```python
from build123d import *

# Parameters (mm, degrees)
SKETCH_1_R          = 3.5
SKETCH_1_R_2        = 3
EXTRUDE_1_DEPTH     = 10
SKETCH_2_R          = 20
EXTRUDE_2_DEPTH     = 16
EXTRUDE_2_DRAFT     = -5
SKETCH_4_W          = 48
SKETCH_4_H          = 48
CUT_EXTRUDE_1_DEPTH = 16
EXTRUDE_3_DEPTH     = 2
EXTRUDE_3_DRAFT     = -10


with BuildPart() as part:
    # Sketch 1 → Extrude 1 (new body)
    with BuildSketch(Plane(origin=(0, 0, 0), x_dir=(1, 0, 0), z_dir=(0, 1, 0))):
        with BuildLine():
            Line((0, -20), (69, -20))
            ThreePointArc((69, -20), (73.242640687, -18.242640687), (75, -14))
            Line((75, -14), (75, 37))
            Line((75, 37), (37, 75))
            Line((37, 75), (-14, 75))
            ThreePointArc((-14, 75), (-18.242640687, 73.242640687), (-20, 69))
            Line((-20, 69), (-20, 0))
            ThreePointArc((-20, 0), (-14.142135624, -14.142135624), (0, -20))
        make_face()
        with Locations(Location((65, -5, 0), (0, 0, 270))):
            Circle(SKETCH_1_R, mode=Mode.SUBTRACT)
        with Locations(Location((55, -10, 0), (0, 0, 270))):
            Circle(SKETCH_1_R_2, mode=Mode.SUBTRACT)
        with Locations(Location((30, -5, 0), (0, 0, 270))):
            Circle(SKETCH_1_R, mode=Mode.SUBTRACT)
        with Locations(Location((25, -10, 0), (0, 0, 270))):
            Circle(SKETCH_1_R_2, mode=Mode.SUBTRACT)
        with Locations(Location((-5, 30, 0), (0, 0, 270))):
            Circle(SKETCH_1_R, mode=Mode.SUBTRACT)
        with Locations(Location((-5, 65, 0), (0, 0, 270))):
            Circle(SKETCH_1_R, mode=Mode.SUBTRACT)
        with Locations(Location((-10, 25, 0), (0, 0, 270))):
            Circle(SKETCH_1_R_2, mode=Mode.SUBTRACT)
        with Locations(Location((-10, 55, 0), (0, 0, 270))):
            Circle(SKETCH_1_R_2, mode=Mode.SUBTRACT)
    extrude(amount=-EXTRUDE_1_DEPTH)


with BuildPart() as extrude_2_tool:
    # Sketch 2 → Extrude 2 (with draft: the straight prism first)
    with BuildSketch(Plane(origin=(0, -10, 0), x_dir=(1, 0, 0), z_dir=(0, 1, 0))):
        Circle(SKETCH_2_R)
    extrude(amount=-EXTRUDE_2_DEPTH)
    # Extrude 2: the draft: its side faces are tilted about the plane it starts from
    extrude_2_sides = [extrude_2_tool.faces().sort_by_distance(p)[0] for p in [
        (-20, -18, 0),
    ]]
    draft(extrude_2_sides, Plane(origin=(0, -10, 0), x_dir=(1, 0, 0), z_dir=(0, 1, 0)), EXTRUDE_2_DRAFT)


with BuildPart() as part_1:
    add(part.part)

    # Extrude 2: add extrude_2_tool
    add(extrude_2_tool.part)

    # Sketch 3 → Revolve 1 (revolve)
    with BuildSketch(Plane.XY, mode=Mode.PRIVATE) as revolve_1_sk:
        Polygon((0, -26), (12, -26), (14.4, -26.643078062), (14.4, -33.356921938), (12, -34), (0, -34), align=None)
    revolve(revolve_1_sk.sketch.rotate(Axis((0, -34, 0), (0, 1, 0)), 270), axis=Axis((0, -34, 0), (0, 1, 0)))

    # Sketch 4 → Cut-Extrude 1 (cut)
    with BuildSketch(Plane(origin=(0, -26, 0), x_dir=(1, 0, 0), z_dir=(0, 1, 0))):
        Rectangle(SKETCH_4_W, SKETCH_4_H)
        Polygon((-12, -6.92820323), (0, -13.856406461), (12, -6.92820323), (12, 6.92820323), (0, 13.856406461), (-12, 6.92820323), align=None, mode=Mode.SUBTRACT)
    extrude(amount=-CUT_EXTRUDE_1_DEPTH, mode=Mode.SUBTRACT)

    # Sketch 5 → Cut-Revolve 1 (revolve, cut)
    with BuildSketch(Plane.XY, mode=Mode.PRIVATE) as cut_revolve_1_sk:
        Polygon((0, 0), (8, 0), (6.9175, -1.0825), (6.9175, -32.9175), (8, -34), (0, -34), align=None)
    revolve(cut_revolve_1_sk.sketch.rotate(Axis((0, -34, 0), (0, 1, 0)), 270), axis=Axis((0, -34, 0), (0, 1, 0)), mode=Mode.SUBTRACT)


with BuildPart() as extrude_3_tool:
    # Sketch 6 → Extrude 3 (with draft: the straight prism first)
    with BuildSketch(Plane(origin=(0, -10, 0), x_dir=(1, 0, 0), z_dir=(0, 1, 0))):
        with BuildLine():
            Line((6.573950263, 34.573950263), (34.573950263, 6.573950263))
            ThreePointArc((34.573950263, 6.573950263), (38.109484168, 5.109484168), (41.645018074, 6.573950263))
            Line((41.645018074, 6.573950263), (69.929289322, 34.85822151))
            ThreePointArc((69.929289322, 34.85822151), (71.393755416, 38.393755416), (69.929289322, 41.929289322))
            Line((69.929289322, 41.929289322), (41.929289322, 69.929289322))
            ThreePointArc((41.929289322, 69.929289322), (38.393755416, 71.393755416), (34.85822151, 69.929289322))
            Line((34.85822151, 69.929289322), (6.573950263, 41.645018074))
            ThreePointArc((6.573950263, 41.645018074), (5.109484168, 38.109484168), (6.573950263, 34.573950263))
        make_face()
    extrude(amount=-EXTRUDE_3_DEPTH)
    # Extrude 3: the draft: its side faces are tilted about the plane it starts from
    extrude_3_sides = [extrude_3_tool.faces().sort_by_distance(p)[0] for p in [
        (20.573950263, -11, -20.573950263),
        (38.109484168, -11, -5.109484168),
        (55.787153698, -11, -20.716085886),
        (71.393755416, -11, -38.393755416),
        (55.929289322, -11, -55.929289322),
        (38.393755416, -11, -71.393755416),
        (20.716085886, -11, -55.787153698),
        (5.109484168, -11, -38.109484168),
    ]]
    draft(extrude_3_sides, Plane(origin=(0, -10, 0), x_dir=(1, 0, 0), z_dir=(0, 1, 0)), EXTRUDE_3_DRAFT)


with BuildPart() as part_2:
    add(part_1.part)

    # Extrude 3: add extrude_3_tool
    add(extrude_3_tool.part)

    # Sketch 7 → Revolve 2 (revolve)
    with BuildSketch(Plane(origin=(0, 0, 0), x_dir=(0.7071067811865476, 0, -0.7071067811865475), z_dir=(0.7071067811865475, 0, 0.7071067811865476)), mode=Mode.PRIVATE) as revolve_2_sk:
        with BuildLine():
            Line((55, -12), (75, -12))
            Line((75, -12), (72.585786438, -14.414213562))
            ThreePointArc((72.585786438, -14.414213562), (71.93693974, -14.847759065), (71.171572875, -15))
            Line((71.171572875, -15), (55, -15))
            Line((55, -15), (55, -12))
        make_face()
    revolve(revolve_2_sk.sketch.rotate(Axis((38.890872965, -15, -38.890872965), (0, 1, 0)), 225), axis=Axis((38.890872965, -15, -38.890872965), (0, 1, 0)))


solid = part_2.part
```
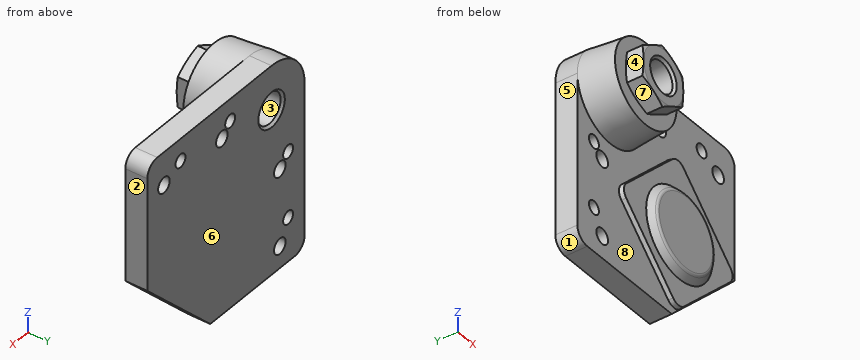
Read the model definition and answer for the solid it produces. Units are mm, in the model's axes. Face numbers are marked on the shaded views. A direction names the side the tool comes from. Round coordinates to 2 decimals unless told otherwise and drop trailing zeros. Loops run counter-clockwise (first coordinate to the right, second up) from the corner with the lowest first, then second, coordinate; pieces in that order, holes last. Notation, with made-up numbers: (14, -6.5) -> (18, -6.5) arc R17 cw to (18, -2.5) -> close; hole circle Ø11 at (75, 36.25). An arc over 180 degrees is marked (long way). One line per item, written item: value.
1) For the marked faces 4, 5, 6, 7 and 8, determine the directions among +Z, -Z, +X, -X, +Y, -Y from which every point of the face is accessible in a straight line to the end or side of a thin tool.
Answer list:
face 4: +Z, -Z, -X, -Y
face 5: +Z, -Z, -X, +Y, -Y
face 6: +Z, -Z, +X, -X, +Y
face 7: -Z, -X, -Y
face 8: -Y
2) A cutting plane is placed at B-B (x = 67). Determine the outline of the cut face in (y, z).
Answer list:
outline: (-12, -44.36) -> (-10, -44.86) -> (-10, -45) -> (0, -45) -> (0, 2.13) -> (-10, 2.13) -> (-10, -31.93) -> (-12, -32.43) -> close; (-10, 7.87) -> (0, 7.87) -> (0, 20) -> (-10, 20) -> close
3) A cutting plane is placed at C-C (x = -10). Give the number of separate pieces and of enclosed holes in the cut face, and give its area (3 significant figures).
Answer list:
separate pieces: 3
enclosed holes: 0
area: 1,460 mm²
4) Consider L1, parallel to X at y = -4.25, z = 5; L2, parallel to X at y = -2.5, z = 3.5; L3, parallel to Y at x = 30, z = -46.5. Determine where each line is inside the solid, lowest interval first. Write a range as [from, to].
Answer list:
L1: x = [-19.36, -4.78], [4.78, 26.5], [33.5, 61.5], [68.5, 75]
L2: x = [-19.69, -5.97], [5.97, 26.84], [33.16, 61.84], [68.16, 75]
L3: y = [-15, 0]
5) The mould has two halves that part along Z. Classify the marked faces 1, 2 and 3: pulls with the +Z half, pulls with the -Z half, needs draft (parallel to the pull), parting line crosses it, or undercut.
Answer list:
face 1: pulls with the -Z half
face 2: needs draft
face 3: undercut
6) A cutting plane is placed at A-A (y = -31). Determine the outline of the cut face in (x, z) (1 decimal), and give its area (4 significant figures).
Answer list:
outline: (-12, -6.9) -> (0, -13.9) -> (12, -6.9) -> (12, 6.9) -> (0, 13.9) -> (-12, 6.9) -> close; hole circle Ø13.8 at (0, 0)
area: 348.5 mm²
7) Flat-ended cylindrical pins translate along their axes: P1, Ø9, axis at y = -31.5, z = 3.5, coming from the -X side; P2, Ø5.5, axis at x = -5, z = -30, coming from the +Y side; P3, Ø6.5, axis at y = -28.5, z = -2, coming from the +X side; P4, Ø8, axis at x = -10, z = -25, coming from the +Y side. Find the tip coordinate at first contact, or state that the pin passes through.
Answer list:
P1: stops at x = -12
P2: passes through
P3: stops at x = 18.63
P4: stops at y = 0
